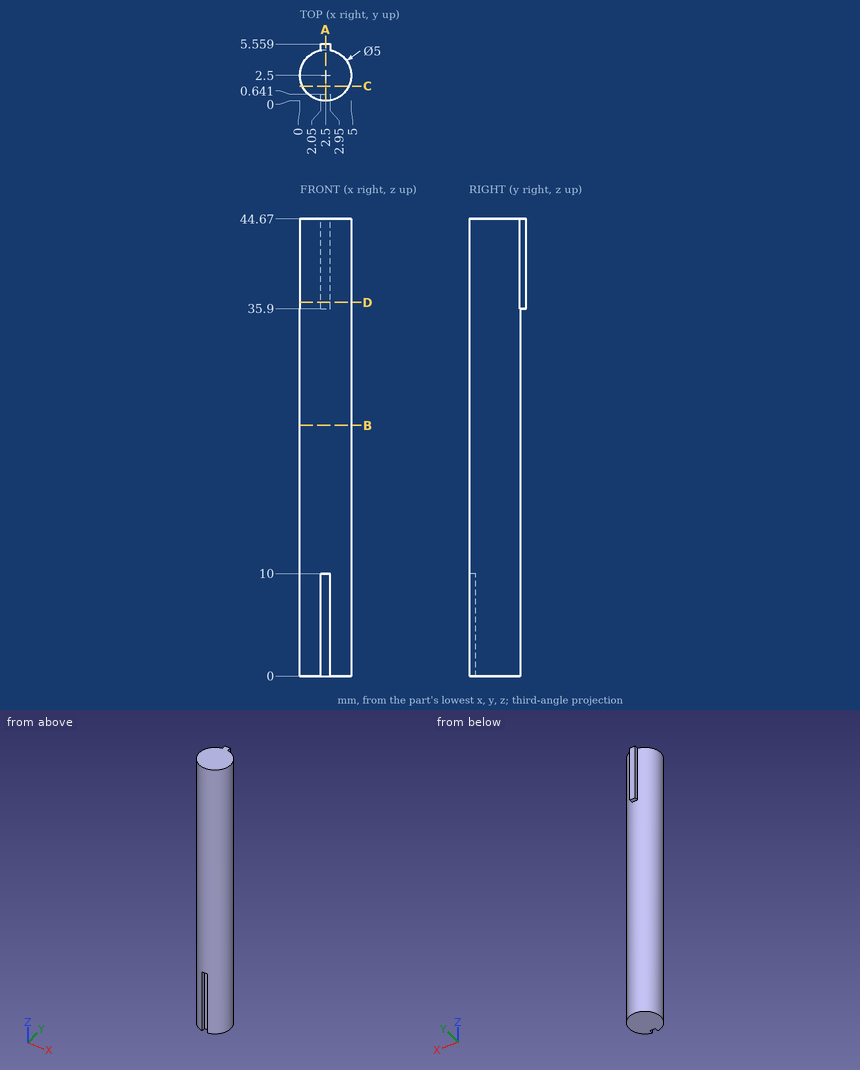
Check sheet for the drawn part. Datum: minimum x, y, z corner. Units: mm. Round coordinates to 2 decimals unless told otherwise and drop trailing zeros. Order: outer loops, then holes, each group sorted by start corner. A loop starts at its lowest first (then second) coordinate and runs counter-clockwise, first axis right, second up. Notation, with made-up numbers: M 77.25,76.25 L 135.25,76.25 A19 ccw 135.25,89.25 Z; hole C -11.75,27.25 d9. An arc over 180 degrees is marked long. Answer in a Markdown table with one row per item.
(1) Section check A-A on x = 2.5. Record the boundary of the cut face in (y, z), plus the area to 3 significant figures.
Findings:
| item | result |
|---|---|
| outline | M 0,10 L 0.64,10 L 0.64,0 L 5,0 L 5,35.9 L 5.56,35.9 L 5.56,44.67 L 0,44.67 Z |
| area | 222 mm^2 |
(2) Gauge pin test, flat ends, axial feed: pin 1 (0.5 mm diameter, centred on y = 5, z = 40.5, fed in from +X); pin 2 (1 mm diameter, centred on x = 1.5, z = 29.5, fed in from -Y); pin 3 (2 mm diameter, centred on x = 2, z = 23.5, fed in from +Y). Record the tip position at first contact, or that the pin passes through.
Findings:
| item | result |
|---|---|
| pin 1 | stops at x = 3.59 |
| pin 2 | stops at y = 0.05 |
| pin 3 | stops at y = 5 |
(3) Section check C-C on y = 1.45. Record the boundary of the cut face in (x, z).
Findings:
| item | result |
|---|---|
| outline | M 0.23,0 L 4.77,0 L 4.77,44.67 L 0.23,44.67 Z |
(4) Material ranges on line 1 along Y through (x, z) = (2.45, 14); line 2 along X through (y, z) = (4.2, 36); line 3 along X through (y, z) = (3.4, 41.5), recorded low to high. Write a range as from..to.
Findings:
| item | result |
|---|---|
| line 1 | y = 0..5 |
| line 2 | x = 0.67..4.33 |
| line 3 | x = 0.17..4.83 |
(5) Section check B-B on z = 24.5. Record the boundary of the cut face in (x, y).
Findings:
| item | result |
|---|---|
| outline | C 2.5,2.5 d5 |
(6) Section check D-D on z = 36.5. Record the boundary of the cut face in (x, y).
Findings:
| item | result |
|---|---|
| outline | M 2.05,4.96 A2.5 ccw long 2.95,4.96 L 2.95,5.56 L 2.05,5.56 Z |
